Check sheet for the modelled part. Datum: model origin and axes. Units: mm. Round coordinates to 2 decimals unless told otherwise and drop trailing zeros. Write each loop counter-clockwise with the first axis right and the second up, starting at its lowest first coordinate (ties: lowest second). Pieces come first, ordered by that corner, then holes. Notation, with made-up numbers: (57, 83.25) -> (70, 83.25) arc R17 cw to (70, 102.25) -> close; hole circle Ø5 at (0, -11). An arc over 180 degrees is marked (long way). Put each result on its own line as item: value. Start each with the question number.
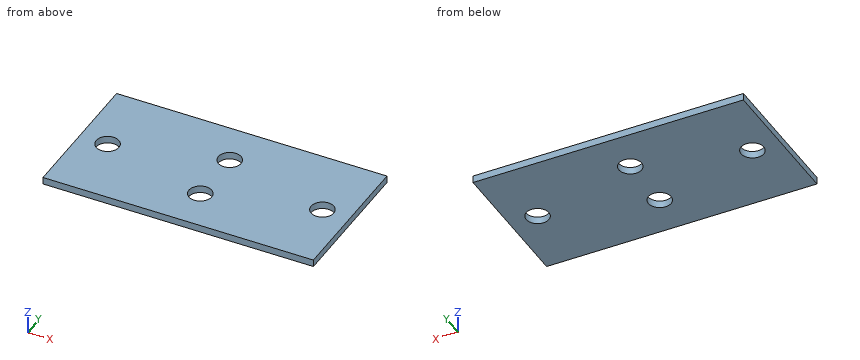
Autodesk Inventor part; units mm, degrees
ref_plane "YZ Plane" through (0, 0, 0) normal (1, 0, 0) x (0, 1, 0)
ref_plane "XZ Plane" through (0, 0, 0) normal (0, 1, 0) x (-1, 0, 0)
ref_plane "XY Plane" through (0, 0, 0) normal (0, 0, 1) x (1, 0, 0)
sketch "Sketch1" plane through (0, 0, 0) normal (0, 0, 1) x (1, 0, 0)
  line L0 (-19, 10) -> (19, 10)
  line L1 (19, 10) -> (19, -10)
  line L2 (19, -10) -> (-19, -10)
  line L3 (-19, -10) -> (-19, 10)
  line L4 (-19, 10) -> (19, -10) construction
  line L5 (19, 10) -> (-19, -10) construction
  circle A0 centre (15.1, 0) radius 1.6
  line L6 (0, 0) -> (12.8976, 0)
  line L7 (0, 0) -> (0, 11.3109)
  circle A1 centre (-15.1, 0) radius 1.6
  circle A2 centre (0, -4) radius 1.6
  circle A3 centre (0, 4) radius 1.6
  dimension "d0" = 38
  dimension "d1" = 20
  dimension "d2" = 3.2
  dimension "d3" = 3.9
  dimension "d17" = 6
  dimension "d18" = 3.2
sketch "Sketch2" plane through (0, 0, 1) normal (0, 0, 1) x (1, 0, 0)
  line L0 (-17.5, 30) -> (-12.5, 30)
  line L1 (-7.5, 25) -> (-7.5, 10)
  line L2 (-12.5, 5) -> (-17.5, 5)
  line L3 (-22.5, 10) -> (-22.5, 25)
  line L4 (-22.5, 30) -> (-7.5, 5) construction
  line L5 (-7.5, 30) -> (-22.5, 5) construction
  line L6 (-28.3073, 0) -> (28.3073, 0)
  line L7 (0, 37.5) -> (0, -37.5)
  arc A0 (-17.5, 30) -> (-22.5, 25) centre (-17.5, 25) ccw
  arc A1 (-7.5, 25) -> (-12.5, 30) centre (-12.5, 25) ccw
  arc A2 (-12.5, 5) -> (-7.5, 10) centre (-12.5, 10) ccw
  arc A3 (-22.5, 10) -> (-17.5, 5) centre (-17.5, 10) ccw
  line L8 (17.5, 30) -> (12.5, 30)
  line L9 (7.5, 25) -> (7.5, 10)
  line L10 (12.5, 5) -> (17.5, 5)
  line L11 (22.5, 10) -> (22.5, 25)
  line L12 (22.5, 30) -> (7.5, 5) construction
  line L13 (7.5, 30) -> (22.5, 5) construction
  arc A4 (22.5, 25) -> (17.5, 30) centre (17.5, 25) ccw
  arc A5 (12.5, 30) -> (7.5, 25) centre (12.5, 25) ccw
  arc A6 (7.5, 10) -> (12.5, 5) centre (12.5, 10) ccw
  arc A7 (17.5, 5) -> (22.5, 10) centre (17.5, 10) ccw
  line L14 (-17.5, -30) -> (-12.5, -30)
  line L15 (-7.5, -25) -> (-7.5, -10)
  line L16 (-12.5, -5) -> (-17.5, -5)
  line L17 (-22.5, -10) -> (-22.5, -25)
  line L18 (-22.5, -30) -> (-7.5, -5) construction
  line L19 (-7.5, -30) -> (-22.5, -5) construction
  arc A8 (-22.5, -25) -> (-17.5, -30) centre (-17.5, -25) ccw
  arc A9 (-12.5, -30) -> (-7.5, -25) centre (-12.5, -25) ccw
  arc A10 (-7.5, -10) -> (-12.5, -5) centre (-12.5, -10) ccw
  arc A11 (-17.5, -5) -> (-22.5, -10) centre (-17.5, -10) ccw
  arc A12 (7.5, -25) -> (12.5, -30) centre (12.5, -25) ccw
  line L20 (7.5, -25) -> (7.5, -10)
  line L21 (17.5, -30) -> (12.5, -30)
  arc A13 (17.5, -30) -> (22.5, -25) centre (17.5, -25) ccw
  arc A14 (12.5, -5) -> (7.5, -10) centre (12.5, -10) ccw
  line L22 (22.5, -10) -> (22.5, -25)
  arc A15 (22.5, -10) -> (17.5, -5) centre (17.5, -10) ccw
  line L23 (7.5, -30) -> (22.5, -5) construction
  line L24 (22.5, -30) -> (7.5, -5) construction
  line L25 (12.5, -5) -> (17.5, -5)
  point P0 (0, 0)
  point P1 (-15, 17.5)
  point P2 (0, 0)
  point P3 (15, 17.5)
  point P4 (-15, -17.5)
  point P5 (15, -17.5)
  dimension "d9" = 15
  dimension "d10" = 25
  dimension "d12" = 10
  dimension "d13" = 15
  dimension "d14" = 5
extrude "Plate1" add sketch "Sketch1" along normal blind 1
equation "\"d5\" = 厚度"
equation "\"折彎半徑\" = 厚度"
equation "\"折彎離隙寬度\" = 厚度"
equation "\"折彎離隙深度\" = 0.5 * 厚度"
equation "\"轉角離隙大小\" = 4 * 厚度"
equation "\"最小剩餘\" = 2 * 厚度"
equation "\"轉移半徑\" = 折彎半徑"
equation "\"Jacobi半徑大小\" = 折彎半徑"
equation "\"間隙大小\" = 厚度"
properties part number "battery_box_5V_side1" material "Aluminum"
1. Section check D-D, the plane x = 15.1. Enter the section's corners in (y, z).
2. Section check B-B, the plane z = 0.75. Enter the section's corners in (x, y).
3. Material ranges on L1, parallel to Y at x = 0, z = 0.4; L2, parallel to X at y = 4, z = 0.4; L3, parallel to X at y = -1, z = 0.3, recorded low to high. Write a range as [from, to].
4. Section check C-C, the plane y = -4. Enter the section's corners in (x, z), then the cut area to 3 significant figures.
5. Gauge pin test, flat end, axial feed: P1, Ø1.9, axis at x = 0, y = -4, coming from the -Z side. Record the tip position at first contact, or that the pin passes through.
6. Section check A-A, the plane x = 0. Enter the section's corners in (y, z), then the cut area to 3 significant figures.
Reply:
1. outline: (-10, 0) -> (-1.6, 0) -> (-1.6, 1) -> (-10, 1) -> close; (1.6, 0) -> (10, 0) -> (10, 1) -> (1.6, 1) -> close
2. outline: (-19, -10) -> (19, -10) -> (19, 10) -> (-19, 10) -> close; hole circle Ø3.2 at (-15.1, 0); hole circle Ø3.2 at (0, -4); hole circle Ø3.2 at (0, 4); hole circle Ø3.2 at (15.1, 0)
3. L1: y = [-10, -5.6], [-2.4, 2.4], [5.6, 10]
3. L2: x = [-19, -1.6], [1.6, 19]
3. L3: x = [-19, -16.35], [-13.85, 13.85], [16.35, 19]
4. outline: (-19, 0) -> (-1.6, 0) -> (-1.6, 1) -> (-19, 1) -> close; (1.6, 0) -> (19, 0) -> (19, 1) -> (1.6, 1) -> close
4. area: 34.8 mm2
5. P1: passes through
6. outline: (-10, 0) -> (-5.6, 0) -> (-5.6, 1) -> (-10, 1) -> close; (-2.4, 0) -> (2.4, 0) -> (2.4, 1) -> (-2.4, 1) -> close; (5.6, 0) -> (10, 0) -> (10, 1) -> (5.6, 1) -> close
6. area: 13.6 mm2
